Source: CAD feature listing. Evaluate the final solid. Frame: model axes, mm. A direction names the side the tool comes from. Round coordinates to 2 decimals unless told otherwise and drop trailing zeros. Write each loop counter-clockwise with the first axis right and the second up, starting at its lowest first coordinate (ties: lowest second). Pieces come first, ordered by that corner, then holes. Notation, with made-up numbers: M 14.5,61.25 L 73.5,61.25 A29 ccw 73.5,92.25 Z; hole C 15,16 d7. An arc over 180 degrees is marked long. Answer in a Markdown table with one row per item. Add a question column.
Item 1: Cut plane D-D on y = -8. Return loops of the section in (x, z).
Item 2: Mould query, pull axis Y, two halves, no side actions, for faces 4 (the face through (-56.055, -0.285, -33.153)), 5 (the face through (-56.055, -19.715, -33.153)), 6 (the face through (-24.356, -10, -20)), 7 (the face through (-50.04, -13.38, -33.15)). Classes: released by +Y, released by -Y, zero draft, split by the parting line, or undercut.
Item 3: Contact query for flat-ended pins moving along their axis: pin 1 (1 mm diameter, centred on x = -25, y = -18, fed in from -Z); pin 2 (6 mm diameter, centred on y = -8.5, z = -10.5, fed in from -X); pin 3 (10 mm diameter, centred on x = -32.5, y = -7.5, fed in from +Z). Output: stop coordinate, or through.
Item 4: Cut plane B-B on x = -49. Return loops of the section in (y, z).
Item 5: Material intervals for probe 1 along Z at (x, y) = (-34, -11.25); probe 2 along X at (y, z) = (-10, -33.4); probe 3 along X at (y, z) = (-3, -27.25), sorted ascending.
Item 6: Set-up query: faces 1 (the face through (-25, -18, -28.139)), 2 (the face through (-26.356, -8, -19)), 3 (the face through (-25, -10, -4.139)). Return all of +Z, -Z, +X, -X, +Y, -Y with unobstructed straight access to the full face (end or side cutting, diameter ignored); none if empty.
Item 7: Cut plane A-A on y = -17. Return loops of the section in (x, z).
Item 8: Cut plane C-C on z = -13. Return loops of the section in (x, y).
from build123d import *

# Parameters (mm, degrees)
F1_DEPTH = 20
F3_DEPTH = 3
F4_R     = 5
F5_DEPTH = 3
F6_R     = 5
F7_DEPTH = 3
F8_R     = 1


with BuildPart() as f1:
    # F0 (on Front) → F1 (new body)
    with BuildSketch(Plane.XZ):
        with BuildLine():
            Line((-29.355609, -32.139022), (-56.355609, -32.139022))
            Line((-56.355609, -32.139022), (-56.355609, -34.139022))
            Line((-56.355609, -34.139022), (-29.355609, -34.139022))
            ThreePointArc((-29.355609, -34.139022), (-25.820076, -32.674556), (-24.355609, -29.139022))
            Line((-24.355609, -29.139022), (-24.355609, -4.139022))
            Line((-24.355609, -4.139022), (-26.355609, -4.139022))
            Line((-26.355609, -4.139022), (-26.355609, -29.139022))
            ThreePointArc((-26.355609, -29.139022), (-27.234289, -31.260342), (-29.355609, -32.139022))
        make_face()
    extrude(amount=F1_DEPTH)

    # F2 (on face) → F3 (cut)
    with BuildSketch(Plane.YZ.offset(-24.355609)):
        Polygon((-17.18655, -24.139022), (-20, -24.139022), (-20, -28.139022), (-15, -28.139022), (-15, -24.139022), align=None)
    extrude(amount=-F3_DEPTH, mode=Mode.SUBTRACT)

    # F4 (on face) → F5 (cut)
    with BuildSketch(Plane.YZ.offset(-24.355609)):
        with Locations((-10, -14.139022)):
            Circle(F4_R)
    extrude(amount=-F5_DEPTH, mode=Mode.SUBTRACT)

    # F6 (on face) → F7 (cut)
    with BuildSketch(Plane(origin=(0, 0, -34.139022), x_dir=(1, 0, 0), z_dir=(0, 0, -1))):
        with Locations((-46.355609, 10)):
            Circle(F6_R)
    extrude(amount=-F7_DEPTH, mode=Mode.SUBTRACT)

    # F8
    f8_edges = [f1.edges().sort_by_distance(p)[0] for p in [
        (-25.355609, -20, -4.139022),
        (-25.355609, 0, -4.139022),
        (-56.355609, -20, -33.139022),
        (-56.355609, 0, -33.139022),
    ]]
    fillet(f8_edges, radius=F8_R)


solid = f1.part
Results below:
| question | item | result |
|---|---|---|
| 1 | outline | M -56.36,-34.14 L -50.94,-34.14 L -50.94,-32.14 L -56.36,-32.14 Z; M -41.77,-34.14 L -29.36,-34.14 A5 ccw -24.36,-29.14 L -24.36,-18.72 L -26.36,-18.72 L -26.36,-29.14 A3 cw -29.36,-32.14 L -41.77,-32.14 Z; M -26.36,-9.56 L -24.36,-9.56 L -24.36,-4.14 L -26.36,-4.14 Z |
| 2 | face 4 | released by +Y |
| 2 | face 5 | released by -Y |
| 2 | face 6 | zero draft |
| 2 | face 7 | undercut |
| 3 | pin 1 | z = -32.32 |
| 3 | pin 2 | x = -26.36 |
| 3 | pin 3 | z = -31.5 |
| 4 | outline | M -20,-34.14 L -14.24,-34.14 L -14.24,-32.14 L -20,-32.14 Z; M -5.76,-34.14 L 0,-34.14 L 0,-32.14 L -5.76,-32.14 Z |
| 5 | probe 1 | -34.14 to -32.14 |
| 5 | probe 2 | -56.36 to -51.36, -41.36 to -26.74 |
| 5 | probe 3 | -26.36 to -24.36 |
| 6 | face 1 | +X, -X, -Y |
| 6 | face 2 | +Z, -X, +Y, -Y |
| 6 | face 3 | +Z, +X, -X, +Y, -Y |
| 7 | outline | M -56.36,-34.14 L -29.36,-34.14 A5 ccw -24.36,-29.14 L -24.36,-28.14 L -26.36,-28.14 L -26.36,-29.14 A3 cw -29.36,-32.14 L -56.36,-32.14 Z; M -26.36,-24.14 L -24.36,-24.14 L -24.36,-4.14 L -26.36,-4.14 Z |
| 8 | outline | M -26.36,-20 L -24.36,-20 L -24.36,-14.87 L -26.36,-14.87 Z; M -26.36,-5.13 L -24.36,-5.13 L -24.36,0 L -26.36,0 Z |
